CAD build for the part. Positions are in the model's coordinates, mm. A direction names the side the tool comes from. Coordinates: 2 decimals unless noted, no trailing zeros. Order: outer loops, then holes, each group sorted by start corner. A loop starts at its lowest first (then second) coordinate and runs counter-clockwise, first axis right, second up. Notation, with made-up numbers: M 75.25,27 L 81.25,27 A8 cw 81.25,33 Z; hole C -10.5,85 d4. An arc over 180 degrees is marked long. Write item = value, one per line.
from build123d import *

# Parameters (mm, degrees)
SKETCH_R                   = 18.5
EXTRUDE001_DEPTH           = 14
EXTRUDE001_PLACEMENT_ANGLE = 90
SKETCH002_W                = 5.018169
SKETCH002_H                = 3
EXTRUDE002_DEPTH           = 5
BOX_W                      = 210
BOX_H                      = 320
BOX_DEPTH                  = 320
CUT001_PLACEMENT_ANGLE     = 90
EXTRUDE_DEPTH              = 5


with BuildPart() as hueco:
    # Sketch → Extrude001 (new body)
    with BuildSketch(Plane.XY):
        with Locations((53.478226, 36.958317)):
            Circle(SKETCH_R)
    extrude(amount=EXTRUDE001_DEPTH)


with BuildPart() as hueco_1:
    # Extrude001 placement: moved
    add(hueco.part.moved(Location((-48, -6, -9.25))).rotate(Axis((-48, -6, -9.25), (1, 0, 0)), EXTRUDE001_PLACEMENT_ANGLE))


with BuildPart() as extrude002:
    # Sketch002 → Extrude002 (new body)
    with BuildSketch(Plane.XZ):
        with Locations((27.509085, -11.5)):
            Rectangle(SKETCH002_W, SKETCH002_H)
    extrude(amount=-EXTRUDE002_DEPTH)


with BuildPart() as cubo:
    # Box → Box (new body)
    with BuildSketch(Plane(origin=(0, -151, -150), x_dir=(1, 0, 0), z_dir=(0, 0, 1))):
        with Locations((105, 160)):
            Rectangle(BOX_W, BOX_H)
    extrude(amount=BOX_DEPTH)


with BuildPart() as cut:
    # Sphere → Sphere (revolve)
    with BuildSketch(Plane.XZ):
        with BuildLine():
            ThreePointArc((0, -150), (150, 0), (0, 150))
            Line((0, 150), (0, -150))
        make_face()
    revolve(axis=Axis((0, 0, 0), (0, 0, 1)))

    # Cut: cut Cubo
    add(cubo.part, mode=Mode.SUBTRACT)


with BuildPart() as cut001:
    # Sphere001 → Sphere001 (revolve)
    with BuildSketch(Plane.XZ):
        with BuildLine():
            ThreePointArc((0, -25), (25, 0), (0, 25))
            Line((0, 25), (0, -25))
        make_face()
    revolve(axis=Axis((0, 0, 0), (0, 0, 1)))

    # Cut001: cut Cut
    add(cut.part, mode=Mode.SUBTRACT)


with BuildPart() as cut001_1:
    # Cut001 placement: moved
    add(cut001.part.moved(Location((10, 0, -13))).rotate(Axis((10, 0, -13), (0, 1, 0)), CUT001_PLACEMENT_ANGLE))


with BuildPart() as base:
    # Sketch001 → Extrude (new body)
    with BuildSketch(Plane.XZ):
        Polygon((0, 0), (25, 0), (25, -3), (30, -3), (30, 5), (-5, 5), (-5, -13), (0, -13), align=None)
    extrude(amount=-EXTRUDE_DEPTH)

    # Fusion: union Cut001
    add(cut001_1.part)

    # Fusion001: union Extrude002
    add(extrude002.part)


with BuildPart() as base_1:
    # Fusion001 placement: moved
    add(base.part.moved(Location((-10, 0, 38))))

    # Cut002: cut hueco
    add(hueco_1.part, mode=Mode.SUBTRACT)


solid = base_1.part
(1) Pin check, flat tips, straight feed: pin 1 Ø5.5 at (x, y) = (7, 2.5) entering from -Z; pin 2 Ø1.5 at (y, z) = (3, 26) entering from -X; pin 3 Ø5 at (x, z) = (-4.5, 21.5) entering from +Y. Stop position of each tip, or through.
Evaluation:
pin_1 = 0.44
pin_2 = -15
pin_3 = 24.79
(2) Pull direction Y, two halves, no side cores. Call faces 5 (the face through (17, 5, 27)), 6 (the face through (1, -20, 19)), 7 (the face through (5, -6, 19)), 8 (the face through (-10, 2, 31)): +Y half, -Y half, draft (parallel to the pull), parting line (faces both ways), or undercut.
Evaluation:
face_5 = +Y half
face_6 = undercut
face_7 = undercut
face_8 = draft
(3) Slice it at B-B, the plane x = -3.5. Write the cut outline in (y, z), then the cut area to 3 significant figures.
Evaluation:
outline = M -24.75,25 A24.75 ccw 24.75,25 L -6,25 L -6,11.53 L -20,11.53 L -20,25 Z; M 0,38 L 5,38 L 5,43 L 0,43 Z
area = 799 mm²
(4) Slice it at C-C, the plane z = 12.5. Write the cut outline in (x, y), then the cut area to 3 significant figures.
Evaluation:
outline = M -5.06,-20 L -5.06,-6 L 16.01,-6 L 16.01,-14.57 A21.65 ccw long 8.29,-20 Z
area = 1,200 mm²
(5) Wall check: line 1 (Y direction, x = 0, z = 24.5) (3 decimals); line 2 (Y direction, x = -1, z = 19); line 3 (Y direction, x = -12, z = 28.5). Give the ranges that are in metal, low to high. Write a range as from..to.
Evaluation:
line_1 = -24.995..-20, -6..24.995
line_2 = -24.25..-20, -6..24.25
line_3 = 0..5
(6) Slice it at D-D, the plane y = -7. Write the cut outline in (x, z).
Evaluation:
outline = M -24,25 A24 ccw 24,25 L 23.78,25 A18.5 cw -12.82,25 Z
(7) Tool access for faces 1 (the face through (-2, 0, 40)), 2 (the face through (-15, 2, 34)), 3 (the face through (17, 2, 35)), 4 (the face through (2, 2, 38)): list every direction of +Z, -Z, +X, -X, +Y, -Y with a clear straight run to the whole face (end or side of a thin tool).
Evaluation:
face_1 = +Z, +X, -X, -Y
face_2 = +Z, -X, +Y, -Y
face_3 = +X, +Y, -Y
face_4 = +Y, -Y
(8) Slice it at A-A, the plane x = 13. Write the cut outline in (y, z), then the cut area to 3 significant figures.
Evaluation:
outline = M -21.35,25 A21.35 ccw -20,17.52 L -20,25 Z; M -15.95,10.81 A21.35 ccw 21.35,25 L -6,25 L -6,10.81 Z; M 0,38 L 5,38 L 5,43 L 0,43 Z
area = 554 mm²
